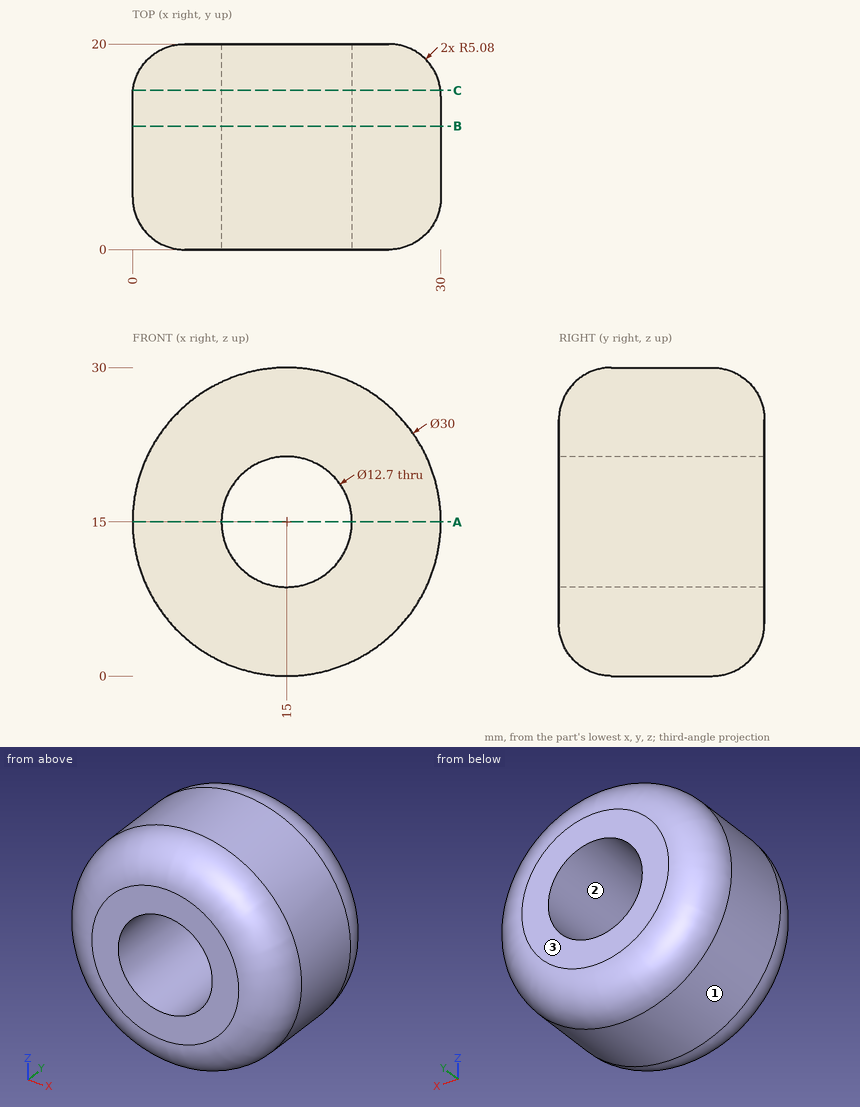
Here's the drawing with two shaded views (mm, measured from the low corner). I have some questions. Coordinates: 2 decimals unless noted, no trailing zeros. Write each loop counter-clockwise with the first axis right and the second up, starting at its lowest first coordinate (ties: lowest second). Pieces come first, ordered by that corner, then holes. Notation, with made-up numbers: (-24.5, -12) -> (11.5, -12) arc R18 cw to (11.5, -1) -> close; hole circle Ø6 at (-5.5, -15.75). An arc over 180 degrees is marked (long way). Use a Markdown table: item, result. Add a question column.
(1) Please list where these lines run through material, in increasing order: line 1 (Z direction, x = 15, y = 9); line 2 (Z direction, x = 15, y = 15.75); line 3 (X direction, y = 3.5, z = 14.5).
(2) If we section it at B-B, the plane y = 12: Write out the boundary of the cut face in (x, z).
(3) If we section it at A-A, the plane z = 15: Write out the boundary of the cut face in (x, y).
(4) We'd pull the mould along X, two halves only. Please class the marked faces 1, 2 and 3: +X half, -X half, draft (parallel to the pull), parting line (faces both ways), or undercut.
(5) If we section it at C-C, the plane y = 15.5: Write out the boundary of the cut face in (x, z).
(6) I'm going to push flat-ended pins straight in: P1, Ø2, axis at y = 5, z = 11.5, coming from the +X side; P2, Ø10, axis at y = 3, z = 9, coming from the +X side; P3, Ø10, axis at x = 15, z = 15, coming from the -Y side; P4, Ø4, axis at x = 9.5, y = 12.5, coming from the -Z side. Where does each tip first touch, or does it pass through?
Outcome:
| question | item | result |
|---|---|---|
| 1 | line 1 | z = 0 to 8.65, 21.35 to 30 |
| 1 | line 2 | z = 0.07 to 8.65, 21.35 to 29.93 |
| 1 | line 3 | x = 0.26 to 8.67, 21.33 to 29.74 |
| 2 | outline | circle Ø30 at (15, 15); hole circle Ø12.7 at (15, 15) |
| 3 | outline | (0, 5.08) arc R5.08 ccw to (5.08, 0) -> (8.65, 0) -> (8.65, 20) -> (5.08, 20) arc R5.08 ccw to (0, 14.92) -> close; (21.35, 0) -> (24.92, 0) arc R5.08 ccw to (30, 5.08) -> (30, 14.92) arc R5.08 ccw to (24.92, 20) -> (21.35, 20) -> close |
| 4 | face 1 | parting line |
| 4 | face 2 | undercut |
| 4 | face 3 | draft |
| 5 | outline | circle Ø29.93 at (15, 15); hole circle Ø12.7 at (15, 15) |
| 6 | P1 | stops at x = 29.79 |
| 6 | P2 | stops at x = 29.93 |
| 6 | P3 | passes through |
| 6 | P4 | stops at z = 0.41 |
